```python
from build123d import *

# Parameters (mm, degrees)
SKETCH1_W           = 65
SKETCH1_H           = 52
BOSS_EXTRUDE1_DEPTH = 1.6
SKETCH2_R           = 1.75
CUT_EXTRUDE1_DEPTH  = 2.6
CHAMFER1_SIZE       = 0.8


with BuildPart() as part:
    # Sketch1 → Boss-Extrude1 (new body)
    with BuildSketch(Plane(origin=(0, 0, 0), x_dir=(1, 0, 0), z_dir=(0, 1, 0))):
        Rectangle(SKETCH1_W, SKETCH1_H)
    extrude(amount=BOSS_EXTRUDE1_DEPTH)

    # Sketch2 → Cut-Extrude1 (cut, through all)
    with BuildSketch(Plane(origin=(0, 1.6, 0), x_dir=(1, 0, 0), z_dir=(0, 1, 0))):
        with Locations((-27.5, -21)):
            Circle(SKETCH2_R)
        with Locations((-27.5, 19)):
            Circle(SKETCH2_R)
        with Locations((27.5, 19)):
            Circle(SKETCH2_R)
        with Locations((27.5, -21)):
            Circle(SKETCH2_R)
    extrude(amount=-CUT_EXTRUDE1_DEPTH, mode=Mode.SUBTRACT)

    # Chamfer1
    chamfer1_edges = [part.edges().sort_by_distance(p)[0] for p in [
        (0, 1.6, 26),
        (0, 1.6, -26),
    ]]
    chamfer(chamfer1_edges, length=CHAMFER1_SIZE)


solid = part.part
```
The model under review builds one solid part; all positions refer to its coordinate system, in mm. Round coordinates to 2 decimals unless told otherwise and drop trailing zeros. Write each loop counter-clockwise with the first axis right and the second up, starting at its lowest first coordinate (ties: lowest second). Pieces come first, ordered by that corner, then holes. Notation, with made-up numbers: (56.25, 86.25) - (78.25, 86.25) arc R25 ccw to (78.25, 110.25) - close; hole circle Ø10 at (39.25, 6.5). An arc over 180 degrees is marked (long way). Use one line per item in the form item = value.
Q1. Consider section C-C (z = 21). State the section outline as (x, y) points.
Answer key:
outline = (-32.5, 0) - (-29.25, 0) - (-29.25, 1.6) - (-32.5, 1.6) - close; (-25.75, 0) - (25.75, 0) - (25.75, 1.6) - (-25.75, 1.6) - close; (29.25, 0) - (32.5, 0) - (32.5, 1.6) - (29.25, 1.6) - close
Q2. Consider section A-A (x = -27.5). State the section outline as (y, z) points, and give its area (3 significant figures).
Answer key:
outline = (0, -26) - (0.8, -26) - (1.6, -25.2) - (1.6, -20.75) - (0, -20.75) - close; (0, -17.25) - (1.6, -17.25) - (1.6, 19.25) - (0, 19.25) - close; (0, 22.75) - (1.6, 22.75) - (1.6, 25.2) - (0.8, 26) - (0, 26) - close
area = 71.4 mm2
Q3. Draft analysis for pull direction X (two halves, no side actions). For faces 1 (the cylindrical face through (26.21, 0.81, -20.18)), 2 (the flat face through (0, 1.6, 0)), 3 (the cylindrical face through (-28.79, 0.81, -20.18)), 4 (the flat face through (-32.5, 1, 0)), state which applies: +X half, -X half, draft (parallel to the pull), parting line (faces both ways), or undercut.
Answer key:
face_1 = undercut
face_2 = draft
face_3 = undercut
face_4 = -X half
Q4. For line 1 (X direction, y = 0.5, z = -19); line 2 (Z direction, x = 27.5, y = 0.65); line 3 (X direction, y = 0.5, z = 22.5), list the stretches that pass through material, from the lowest coordinate up. Write a range as [from, to].
Answer key:
line_1 = [-32.5, -29.25], [-25.75, 25.75], [29.25, 32.5]
line_2 = [-26, -20.75], [-17.25, 19.25], [22.75, 26]
line_3 = [-32.5, -28.4], [-26.6, 26.6], [28.4, 32.5]
Q5. Insertion check: pin 1 Ø3 at (x, z) = (-27.5, 21) entering from -Y. The pin has a flat end and moves straight along its axis. Give the tip position at first contact, or say it passes through.
Answer key:
pin_1 = through
Q6. Consider section B-B (y = 1.05). State the section outline as (x, z) points.
Answer key:
outline = (-32.5, -25.75) - (32.5, -25.75) - (32.5, 25.75) - (-32.5, 25.75) - close; hole circle Ø3.5 at (-27.5, -19); hole circle Ø3.5 at (-27.5, 21); hole circle Ø3.5 at (27.5, -19); hole circle Ø3.5 at (27.5, 21)
